Geometry: final body of the model. Coordinates: model frame, mm. A direction names the side the tool comes from. Coordinates: 2 decimals unless noted, no trailing zeros. Order: outer loops, then holes, each group sorted by start corner. A loop starts at its lowest first (then second) coordinate and runs counter-clockwise, first axis right, second up. Notation, with made-up numbers: M -10.75,20.5 L 48.25,20.5 A11 cw 48.25,35.5 Z; hole C 33.5,32 d6. An arc over 180 degrees is marked long. One line per question, with ' | ' between items.
from build123d import *

# Parameters (mm, degrees)
ESQUISSE1_W             = 52
ESQUISSE1_H             = 140
BOSS_EXTRU_1_DEPTH      = 3
ESQUISSE2_R             = 1
ESQUISSE2_W             = 9
ESQUISSE2_H             = 6
ESQUISSE2_W_2           = 10
ESQUISSE2_W_3           = 6
ESQUISSE2_H_2           = 22
ESQUISSE2_H_3           = 27.999999716
ENL_V_MAT_EXTRU_1_DEPTH = 108.616004474


with BuildPart() as part:
    # Esquisse1 → Boss.-Extru.1 (new body)
    with BuildSketch(Plane.XY):
        with Locations((20.753246753, 26.883116883)):
            Rectangle(ESQUISSE1_W, ESQUISSE1_H)
    extrude(amount=BOSS_EXTRU_1_DEPTH)

    # Esquisse2 → Enlèv. mat.-Extru.1 (cut, through all)
    with BuildSketch(Plane.XY.offset(3)):
        with Locations((3.753246753, -35.116883117)):
            Circle(ESQUISSE2_R)
        with Locations((-0.746753247, 93.883116883)):
            Rectangle(ESQUISSE2_W, ESQUISSE2_H)
        with Locations((20.753246753, 93.883116883)):
            Rectangle(ESQUISSE2_W_2, ESQUISSE2_H)
        Polygon((37.753246753, 96.883116883), (37.753246753, 90.883116883), (40.753246753, 90.883116883), (40.753246753, 82.883116599), (46.753246753, 82.883116599), (46.753246753, 96.883116883), align=None)
        with Locations((43.753246753, 53.883116599)):
            Rectangle(ESQUISSE2_W_3, ESQUISSE2_H_2)
        with Locations((43.753246753, 13.883116599)):
            Rectangle(ESQUISSE2_W_3, ESQUISSE2_H_2)
        with Locations((43.753246753, -29.116883259)):
            Rectangle(ESQUISSE2_W_3, ESQUISSE2_H_3)
    extrude(amount=-ENL_V_MAT_EXTRU_1_DEPTH, mode=Mode.SUBTRACT)


solid = part.part
1. Access query for faces 1 (the face through (44, 24.883, 2)), 2 (the face through (15.753, 94, 2)), 3 (the face through (40.753, 87, 2)). Directions: +Z, -Z, +X, -X, +Y, -Y. A direction counts if a zero-diameter tool reaches every point of the face in a straight line with its end or side. Return the directions, or none.
Response values:
face 1: +Z, -Z, +X | face 2: +Z, -Z, +Y | face 3: +Z, -Z, +X, +Y
2. Material intervals for line 1 (Y direction, x = 44, z = 2.2); line 2 (X direction, y = 87, z = 0.55); line 3 (Y direction, x = 1.5, z = 0.3), sorted ascending. Write a range as [from, to].
Response values:
line 1: y = [-15.12, 2.88], [24.88, 42.88], [64.88, 82.88] | line 2: x = [-5.25, 40.75] | line 3: y = [-43.12, 90.88]
3. Section A-A, the plane z = 1.85. Output: boundary loops of the cut face in (x, y), and give its area (3 significant figures).
Response values:
outline: M -5.25,-43.12 L 40.75,-43.12 L 40.75,-15.12 L 46.75,-15.12 L 46.75,2.88 L 40.75,2.88 L 40.75,24.88 L 46.75,24.88 L 46.75,42.88 L 40.75,42.88 L 40.75,64.88 L 46.75,64.88 L 46.75,82.88 L 40.75,82.88 L 40.75,90.88 L 37.75,90.88 L 37.75,96.88 L 25.75,96.88 L 25.75,90.88 L 15.75,90.88 L 15.75,96.88 L 3.75,96.88 L 3.75,90.88 L -5.25,90.88 Z; hole C 3.75,-35.12 d2 | area: 6,630 mm^2
4. Section C-C, the plane y = 50. Output: boundary loops of the cut face in (x, z).
Response values:
outline: M -5.25,0 L 40.75,0 L 40.75,3 L -5.25,3 Z
5. Pin query (flat end, axial travel): P1, Ø0.9, axis at y = -35.5, z = 2, coming from the +X side; P2, Ø0.9, axis at y = 94, z = 1, coming from the +X side; P3, Ø0.9, axis at x = 19.5, z = 2, coming from the +Y side. Return the tip coordinate at first contact, or that it passes through.
Response values:
P1: stops at x = 40.75 | P2: stops at x = 37.75 | P3: stops at y = 90.88
6. Section B-B, the plane x = 22. Output: boundary loops of the cut face in (y, z), and give its area (3 significant figures).
Response values:
outline: M -43.12,0 L 90.88,0 L 90.88,3 L -43.12,3 Z | area: 402 mm^2
7. Draft query along Y for faces 4 (the face through (17, -43.117, 1)), 5 (the face through (-1, 90.883, 2)), 6 (the face through (44, 64.883, 2)). Return one class per face: pulls with the +Y half, pulls with the -Y half, needs draft (parallel to the pull), parting line crosses it, or undercut.
Response values:
face 4: pulls with the -Y half | face 5: pulls with the +Y half | face 6: undercut
